Could you check a few things on this drawing? It's one solid part, dimensions in mm from its lowest x, y, z. A direction names the side the tool comes from. Give positions to 0.01 mm unless a question says otherwise; leave off trailing zeros. Loops run counter-clockwise (first coordinate to the right, second up) from the corner with the lowest first, then second, coordinate; pieces in that order, holes last. Notation, with made-up numbers: (-31, 82) - (10, 82) arc R31 cw to (10, 113) - close; hole circle Ø5 at (-26, 69). An arc over 180 degrees is marked (long way). Put each result on its own line as item: value. Start each with the question number.
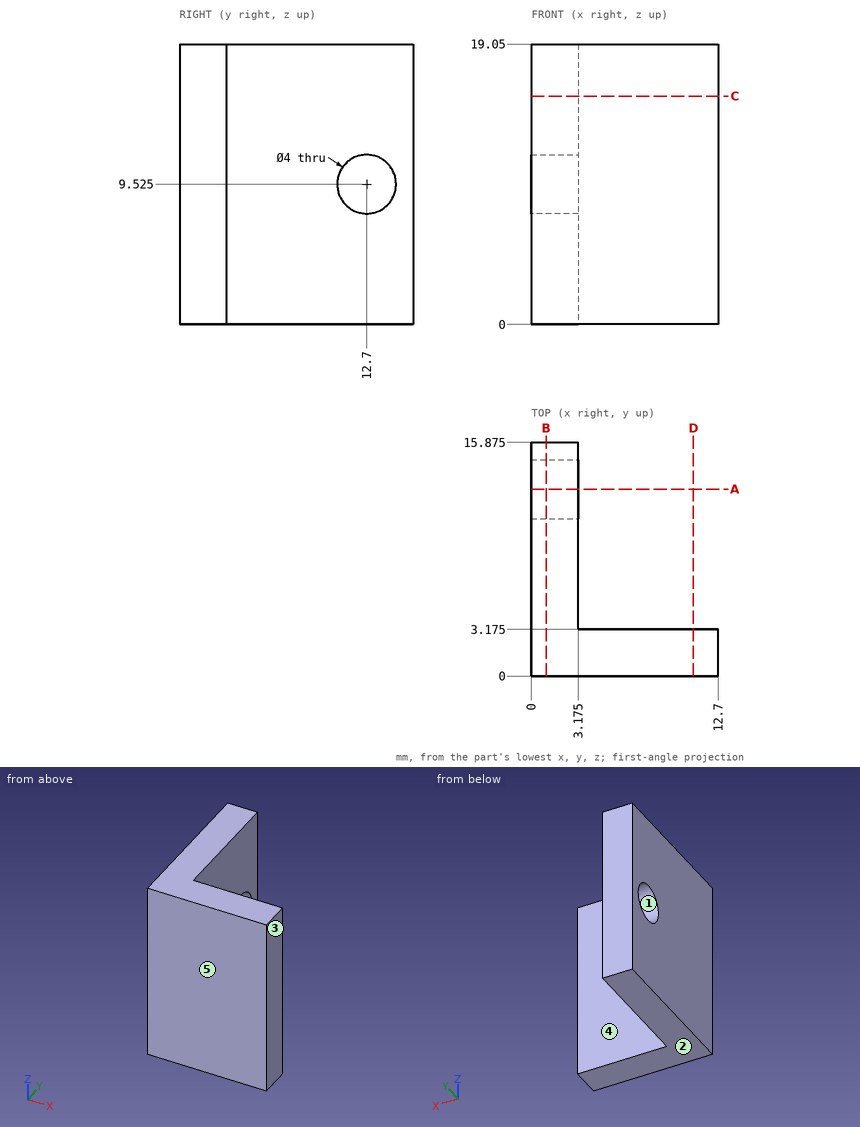
1) Suppose I cut it at B-B on x = 1. Please give me the cut outline in (y, z) (3 decimals).
2) I'm going to push flat-ended pins straight in: P1, Ø2, axis at y = 6.5, z = 13.5, coming from the -X side; P2, Ø4, axis at x = 6.5, y = 10, coming from the +Z side; P3, Ø5, axis at x = 9.5, z = 11, coming from the +Y side (3 decimals). Where does each tip first touch, or does it pass through?
3) Thinking about a two-plate mould opening in Z: for the marked faces 1, 2 and 3, which applies, pulls with the +Z half, pulls with the -Z half, needs draft (parallel to the pull), parting line crosses it, or undercut?
4) Suppose I cut it at C-C on z = 15.5. Please give me the cut outline in (x, y) (3 decimals).
5) Suppose I cut it at D-D on x = 11. Please give me the cut outline in (y, z) (3 decimals).
6) Which directions (+Z, -Z, +X, -X, +Y, -Y) give clear straight access to the entire face, cutting with the end or side of a thin tool? Please do the marked faces 4 and 5.
7) I need wall thicknesses on line 1 (Y direction, x = 8.75, z = 14.5) (3 decimals). Which ranges of the line are inside material? Lowest first, please.
8) Suppose I cut it at A-A on y = 12.7. Please give me the cut outline in (x, z) (3 decimals).
Ans:
1. outline: (0, 0) - (15.875, 0) - (15.875, 19.05) - (0, 19.05) - close; hole circle Ø4 at (12.7, 9.525)
2. P1: stops at x = 0
2. P2: passes through
2. P3: stops at y = 3.175
3. face 1: undercut
3. face 2: pulls with the -Z half
3. face 3: needs draft
4. outline: (0, 0) - (12.7, 0) - (12.7, 3.175) - (3.175, 3.175) - (3.175, 15.875) - (0, 15.875) - close
5. outline: (0, 0) - (3.175, 0) - (3.175, 19.05) - (0, 19.05) - close
6. face 4: +Z, -Z, +X, +Y
6. face 5: +Z, -Z, +X, -X, -Y
7. line 1: y = 0 to 3.175
8. outline: (0, 0) - (3.175, 0) - (3.175, 7.525) - (0, 7.525) - close; (0, 11.525) - (3.175, 11.525) - (3.175, 19.05) - (0, 19.05) - close
